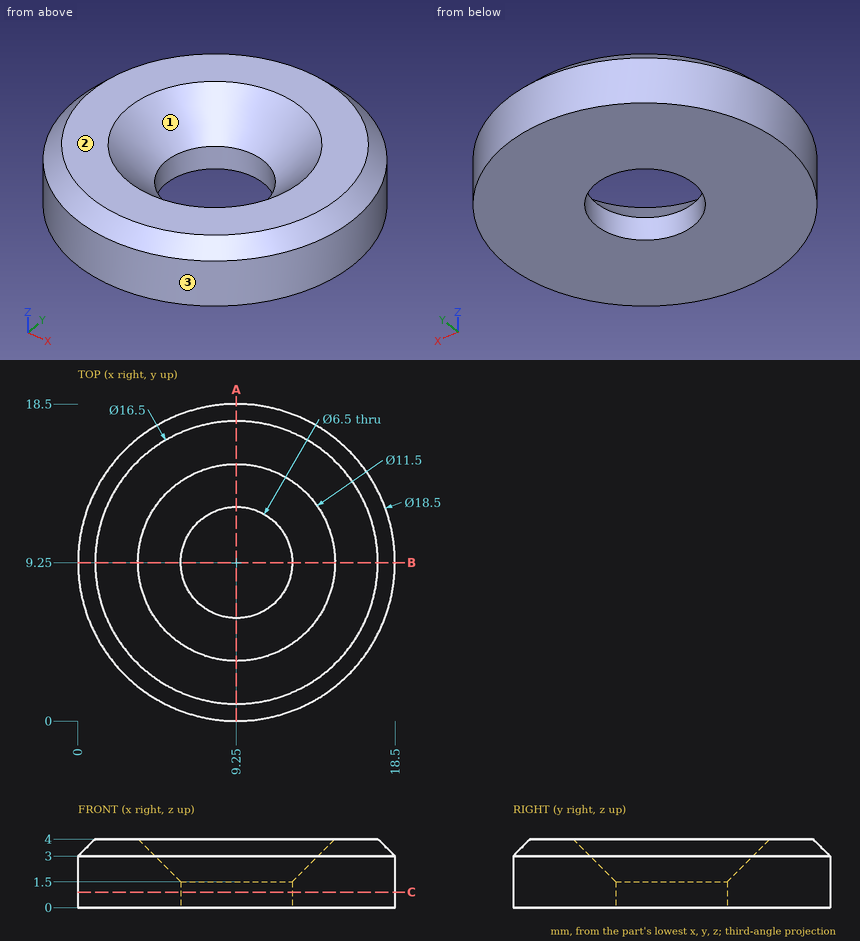
Geometry: see drawing. Coordinates: mm, zero at the bounding-box minimum. Give positions to 0.01 mm unless a question says otherwise; leave off trailing zeros. Write each loop counter-clockwise with the first axis right and the second up, starting at its lowest first coordinate (ties: lowest second). Pieces come first, ordered by that corner, then holes. Notation, with made-up numbers: M 78,56.5 L 101,56.5 A34 ccw 101,93.5 Z; hole C -12.5,49.25 d5. An arc over 180 degrees is marked long. Return JSON: item names as keys, results as strings. Group by question number.
1) Draft query along Y for the marked faces 1, 2 and 3. Return one class per face: released by +Y, released by -Y, zero draft, split by the parting line, or undercut.
2) Cut plane A-A, the plane x = 9.25. Output: boundary loops of the cut face in (y, z).
3) Cut plane C-C, the plane z = 0.9. Output: boundary loops of the cut face in (x, y).
4) Ray query, L1, parallel to Y at x = 9.25, z = 1.25; L2, parallel to X at y = 8.5, z = 3.6; L3, parallel to Y at x = 10.5, z = 3.2. Return the intervals inside material, ascending.
5) First-contact query: pin 1 Ø2 at (x, y) = (13.5, 2) entering from -Z; pin 2 Ø2 at (y, z) = (11.5, 1) entering from +X; pin 3 Ø2 at (y, z) = (12.5, 3) entering from +X; pin 4 Ø1.5 at (x, z) = (13, 3.5) entering from -Y. Flat tips, straight axial feed; report the tip coordinate or a pass-through.
Data:
{
 "1": {"face 1": "undercut", "face 2": "zero draft", "face 3": "split by the parting line"},
 "2": {"outline": "M 0,0 L 6,0 L 6,1.5 L 3.5,4 L 1,4 L 0,3 Z; M 12.5,0 L 18.5,0 L 18.5,3 L 17.5,4 L 15,4 L 12.5,1.5 Z"},
 "3": {"outline": "C 9.25,9.25 d18.5; hole C 9.25,9.25 d6.5"},
 "4": {"L1": "y = 0 to 6, 12.5 to 18.5", "L2": "x = 0.63 to 3.95, 14.55 to 17.87", "L3": "y = 0.29 to 4.46, 14.04 to 18.21"},
 "5": {"pin 1": "stops at z = 0", "pin 2": "stops at x = 18.42", "pin 3": "stops at x = 18.22", "pin 4": "stops at y = 0.57"}
}
